from build123d import *

# Parameters (mm, degrees)
SKETCH1_W                       = 120
SKETCH1_H                       = 110
BOSS_EXTRUDE1_DEPTH             = 3
SKETCH2_W                       = 112
SKETCH2_H                       = 86
BOSS_EXTRUDE2_DEPTH             = 40
BOSS_EXTRUDE3_DEPTH             = 10
BOSS_EXTRUDE3_DEPTH_BACK        = 130
SKIZZE2_R                       = 2
AUFSATZ_LINEAR_AUSTRAGEN1_DEPTH = 3
SKIZZE3_W                       = 3
SKIZZE3_H                       = 30
SCHNITT_LINEAR_AUSTRAGEN1_DEPTH = 13
SKIZZE8_W                       = 3
SKIZZE8_H                       = 30
SCHNITT_LINEAR_AUSTRAGEN2_DEPTH = 13
SKIZZE10_W                      = 80
SKIZZE10_H                      = 2
SCHNITT_LINEAR_AUSTRAGEN3_DEPTH = 1
SKIZZE11_W                      = 80
SKIZZE11_H                      = 2
SCHNITT_LINEAR_AUSTRAGEN4_DEPTH = 1
SKIZZE12_W                      = 55
SKIZZE12_H                      = 10
SCHNITT_LINEAR_AUSTRAGEN5_DEPTH = 31


with BuildPart() as part:
    # Sketch1 → Boss-Extrude1 (new body)
    with BuildSketch(Plane(origin=(0, 0, 0), x_dir=(1, 0, 0), z_dir=(0, 1, 0))):
        with Locations((22.161290323, 12.956989247)):
            Rectangle(SKETCH1_W, SKETCH1_H)
    extrude(amount=BOSS_EXTRUDE1_DEPTH)

    # Sketch2 → Boss-Extrude2 (add)
    with BuildSketch(Plane(origin=(0, 3, 0), x_dir=(1, 0, 0), z_dir=(0, 1, 0))):
        Polygon((-37.838709677, 67.956989247), (-37.838709677, -42.043010753), (-35.838709677, -42.043010753), (-35.838709677, -22.043010753), (80.161290323, -22.043010753), (80.161290323, -42.043010753), (82.161290323, -42.043010753), (82.161290323, 67.956989247), align=None)
        with Locations((22.161290323, 22.956989247)):
            Rectangle(SKETCH2_W, SKETCH2_H, mode=Mode.SUBTRACT)
    extrude(amount=BOSS_EXTRUDE2_DEPTH)

    # Sketch3 → Boss-Extrude3 (add, two sides: drawn at the far end of the back side and taken through both)
    with BuildSketch(Plane(origin=(82.161290323, 0, 0), x_dir=(0, 0, -1), z_dir=(1, 0, 0)).offset(-BOSS_EXTRUDE3_DEPTH_BACK)):
        Polygon((67.956989247, 50), (82.956989247, 0), (67.956989247, 0), align=None)
    extrude(amount=BOSS_EXTRUDE3_DEPTH + BOSS_EXTRUDE3_DEPTH_BACK)

    # Skizze2 → Aufsatz-Linear austragen1 (add)
    # profile 1 of 2: a face of its own
    with BuildSketch(Plane.XZ):
        with BuildLine():
            Line((82.161290323, -67.956989247), (92.161290323, -67.956989247))
            Line((92.161290323, -67.956989247), (92.161290323, -62.956989247))
            ThreePointArc((92.161290323, -62.956989247), (90.696824229, -59.421455341), (87.161290323, -57.956989247))
            Line((87.161290323, -57.956989247), (82.161290323, -57.956989247))
            Line((82.161290323, -57.956989247), (82.161290323, -67.956989247))
        make_face()
        with Locations(Location((87.161290323, -62.956989247, 0), (0, 0, 270))):
            Circle(SKIZZE2_R, mode=Mode.SUBTRACT)
    # profile 2 of 2: a face of its own
    with BuildSketch(Plane.XZ):
        with BuildLine():
            Line((-37.838709677, -67.956989247), (-47.838709677, -67.956989247))
            Line((-47.838709677, -67.956989247), (-47.838709677, -62.956989247))
            ThreePointArc((-47.838709677, -62.956989247), (-46.374243583, -59.421455341), (-42.838709677, -57.956989247))
            Line((-42.838709677, -57.956989247), (-37.838709677, -57.956989247))
            Line((-37.838709677, -57.956989247), (-37.838709677, -67.956989247))
        make_face()
        with Locations(Location((-42.838709677, -62.956989247, 0), (0, 0, 270))):
            Circle(SKIZZE2_R, mode=Mode.SUBTRACT)
    extrude(amount=-AUFSATZ_LINEAR_AUSTRAGEN1_DEPTH)

    # Skizze3 → Schnitt-Linear austragen1 (cut, along a direction that is not the sketch's normal)
    with BuildSketch(Plane(origin=(82.161290323, 0, 0), x_dir=(0, 0, -1), z_dir=(1, 0, 0))):
        with Locations((51.456989247, 22.5)):
            Rectangle(SKIZZE3_W, SKIZZE3_H)
        with Locations((44.456989247, 22.5)):
            Rectangle(SKIZZE3_W, SKIZZE3_H)
        with Locations((37.456989247, 22.5)):
            Rectangle(SKIZZE3_W, SKIZZE3_H)
        with Locations((30.456989247, 22.5)):
            Rectangle(SKIZZE3_W, SKIZZE3_H)
        with Locations((23.456989247, 22.5)):
            Rectangle(SKIZZE3_W, SKIZZE3_H)
        with Locations((16.456989247, 22.5)):
            Rectangle(SKIZZE3_W, SKIZZE3_H)
        with Locations((9.456989247, 22.5)):
            Rectangle(SKIZZE3_W, SKIZZE3_H)
        with Locations((2.456989247, 22.5)):
            Rectangle(SKIZZE3_W, SKIZZE3_H)
    extrude(amount=-SCHNITT_LINEAR_AUSTRAGEN1_DEPTH, dir=(0.7071067811865519, 0, 0.7071067811865432), mode=Mode.SUBTRACT)

    # Skizze8 → Schnitt-Linear austragen2 (cut, along a direction that is not the sketch's normal)
    with BuildSketch(Plane.ZY.offset(37.838709677)):
        with Locations((-51.456989247, 22.5)):
            Rectangle(SKIZZE8_W, SKIZZE8_H)
        with Locations((-44.456989247, 22.5)):
            Rectangle(SKIZZE8_W, SKIZZE8_H)
        with Locations((-37.456989247, 22.5)):
            Rectangle(SKIZZE8_W, SKIZZE8_H)
        with Locations((-30.456989247, 22.5)):
            Rectangle(SKIZZE8_W, SKIZZE8_H)
        with Locations((-23.456989247, 22.5)):
            Rectangle(SKIZZE8_W, SKIZZE8_H)
        with Locations((-16.456989247, 22.5)):
            Rectangle(SKIZZE8_W, SKIZZE8_H)
        with Locations((-9.456989247, 22.5)):
            Rectangle(SKIZZE8_W, SKIZZE8_H)
        with Locations((-2.456989247, 22.5)):
            Rectangle(SKIZZE8_W, SKIZZE8_H)
    extrude(amount=-SCHNITT_LINEAR_AUSTRAGEN2_DEPTH, dir=(-0.7071067811865462, 0, 0.7071067811865488), mode=Mode.SUBTRACT)

    # Skizze10 → Schnitt-Linear austragen3 (cut)
    with BuildSketch(Plane(origin=(-33.838709677, 0, 0), x_dir=(0, 0, -1), z_dir=(1, 0, 0))):
        with Locations((22.956989247, 39)):
            Rectangle(SKIZZE10_W, SKIZZE10_H)
    extrude(amount=-SCHNITT_LINEAR_AUSTRAGEN3_DEPTH, mode=Mode.SUBTRACT)

    # Skizze11 → Schnitt-Linear austragen4 (cut)
    with BuildSketch(Plane.ZY.offset(-78.161290323)):
        with Locations((-22.956989247, 39)):
            Rectangle(SKIZZE11_W, SKIZZE11_H)
    extrude(amount=-SCHNITT_LINEAR_AUSTRAGEN4_DEPTH, mode=Mode.SUBTRACT)

    # Skizze12 → Schnitt-Linear austragen5 (cut)
    with BuildSketch(Plane.XY.offset(22.043010753)):
        with Locations((47.661290323, 12)):
            Rectangle(SKIZZE12_W, SKIZZE12_H)
    extrude(amount=-SCHNITT_LINEAR_AUSTRAGEN5_DEPTH, mode=Mode.SUBTRACT)


solid = part.part
Model file for the job. Use its own axes, mm. A direction names the side the tool comes from. Coordinates: 2 decimals unless noted, no trailing zeros. Order: outer loops, then holes, each group sorted by start corner. A loop starts at its lowest first (then second) coordinate and runs counter-clockwise, first axis right, second up. Notation, with made-up numbers: M 70,-30.75 L 103,-30.75 A26 ccw 103,-7.75 Z; hole C 36.5,87 d1. An arc over 180 degrees is marked long. Return JSON: item names as keys, results as strings.
1. Flat gauge pins, fed straight in: pin 1 (4.5 mm diameter, centred on x = 79.5, z = -19, fed in from +Y); pin 2 (10 mm diameter, centred on x = 30, z = 6, fed in from +Y); pin 3 (2 mm diameter, centred on x = 81, z = -34, fed in from -Y); pin 4 (20 mm diameter, centred on x = 34, y = 16, fed in from -Z). Where does each tip first touch, or does it go through?
Ans:
{"pin 1": "y = 43", "pin 2": "y = 3", "pin 3": "y = 0", "pin 4": "z = -81.16"}
2. Saw through at A-A (x = 60.5). Give the cut face in (y, z), and give its area (3 significant figures).
Ans:
{"outline": "M 0,-82.96 L 50,-67.96 L 43,-67.96 L 43,-65.96 L 3,-65.96 L 3,20.04 L 7,20.04 L 7,22.04 L 3,22.04 L 3,42.04 L 0,42.04 Z; M 17,20.04 L 43,20.04 L 43,22.04 L 17,22.04 Z", "area": "845 mm^2"}
3. Saw through at C-C (x = -22). Give the cut face in (y, z), and give its area (3 significant figures).
Ans:
{"outline": "M 0,-82.96 L 50,-67.96 L 43,-67.96 L 43,-65.96 L 3,-65.96 L 3,20.04 L 43,20.04 L 43,22.04 L 3,22.04 L 3,42.04 L 0,42.04 Z", "area": "865 mm^2"}
4. Tool access for faces 1 (the face through (-42.77, 3, -65.11)), 2 (the face through (85, 1, -57.957)), 3 (the face through (-35.867, 22.29, -40.929)), 4 (the face through (88.85, 1.48, -64.03)): list every direction of +Z, -Z, +X, -X, +Y, -Y with a clear straight run to the whole face (end or side of a thin tool).
Ans:
{"face 1": "+Z, -X, +Y", "face 2": "+Z, +X, +Y, -Y", "face 3": "none", "face 4": "+Y, -Y"}
5. Saw through at D-D (y = 35.5). Give the number of separate pieces and of enclosed holes in the cut face, and give its area (4 significant figures).
Ans:
{"separate pieces": "16", "enclosed holes": "0", "area": "1,665 mm^2"}
6. Drill centre lines: probe 1 along X at (y, z) = (4.5, -39); probe 2 along Y at (x, z) = (50, -58); probe 3 along X at (y, z) = (38.5, 26). Where is each one in solid material? Low to high.
Ans:
{"probe 1": "-37.84 to -33.84, 78.16 to 82.16", "probe 2": "0 to 3", "probe 3": "-37.84 to -35.84, 80.16 to 82.16"}
7. Saw through at B-B (z = 4). Give the cut face in (x, y), and give its area (3 significant figures).
Ans:
{"outline": "M -37.84,0 L 82.16,0 L 82.16,43 L 78.16,43 L 78.16,40 L 79.16,40 L 79.16,38 L 78.16,38 L 78.16,3 L -33.84,3 L -33.84,38 L -34.84,38 L -34.84,40 L -33.84,40 L -33.84,43 L -37.84,43 Z", "area": "676 mm^2"}
8. Pull direction Z, two halves, no side cores. Call faces 5 (the face through (21, 0, -20)), 6 (the face through (4, 2, 42.043)), 7 (the face through (21, 3, -24)): +Z half, -Z half, draft (parallel to the pull), parting line (faces both ways), or undercut.
Ans:
{"face 5": "draft", "face 6": "+Z half", "face 7": "undercut"}
